from build123d import *

# Parameters (mm, degrees)
EXTRUDE_THIN1_DEPTH      = 3
EXTRUDE_THIN1_DEPTH_BACK = 3


with BuildPart() as part:
    # Sketch2 → Extrude-Thin1 (new, two sides)
    with BuildSketch(Plane.XY) as extrude_thin1_sk:
        with BuildLine():
            Line((-42.218873031, 27.812367004), (-33.426518735, 69.811728506))
            ThreePointArc((-33.426518735, 69.811728506), (7.206095545, 85.551006884), (5.054820151, 42.029676007))
            Line((5.054820151, 42.029676007), (-32.043042704, 20.465807333))
            ThreePointArc((-32.043042704, 20.465807333), (-39.516230782, 20.835209769), (-42.218873031, 27.812367004))
        make_face()
        with BuildLine():
            Line((-41.240090772, 27.60746388), (-32.447736476, 69.606825381))
            ThreePointArc((-32.447736476, 69.606825381), (6.620743822, 84.740227406), (4.552280795, 42.894230341))
            Line((4.552280795, 42.894230341), (-32.54558206, 21.330361667))
            ThreePointArc((-32.54558206, 21.330361667), (-38.93087906, 21.645989246), (-41.240090772, 27.60746388))
        make_face(mode=Mode.SUBTRACT)
    extrude(amount=EXTRUDE_THIN1_DEPTH)
    extrude(extrude_thin1_sk.sketch, amount=-EXTRUDE_THIN1_DEPTH_BACK)


solid = part.part
The model under review builds one solid part; all positions refer to its coordinate system, in mm. A direction names the side the tool comes from. Round coordinates to 2 decimals unless told otherwise and drop trailing zeros. Order: outer loops, then holes, each group sorted by start corner. A loop starts at its lowest first (then second) coordinate and runs counter-clockwise, first axis right, second up. Notation, with made-up numbers: (26.5, 76) -> (42.5, 76) arc R32 ccw to (42.5, 113) -> close; hole circle Ø10 at (54.5, -38). An arc over 180 degrees is marked (long way). Write item = value, one per line. Start each with the question number.
Item 1: Consider section A-A on y = 51. Write out the cut boundary in (x, z), plus the area to 3 significant figures.
Item 2: Mouldability with a two-part tool opening along Y and no side actions: class faces 3 (the face through (-13.23, 31.4, 0.04)), 4 (the face through (-1, 39, -3)), 5 (the face through (-13.74, 32.26, 0.04)) as released by +Y, released by -Y, zero draft, split by the parting line, or undercut.
Item 3: Consider section C-C on z = 1.85. Write out the cut boundary in (x, y).
Item 4: For line 1 along X through (y, z) = (76.5, -1.3); line 2 along Y through (x, z) = (-19, -2.35); line 3 along Y through (x, z) = (-8, -1.2), list the stretches that pass through material, from the lowest coordinate up.
Item 5: For faces 1 (the face through (-37.884, 48.518, 0.042)), 2 (the face through (-36.905, 48.313, 0.042)), list the 3-axis set-ups (+Z, -Z, +X, -X, +Y, -Y) from which the entire face can be reached by the end or side of a thin tool; tool diameter is ignored.
Item 6: Consider section B-B on x = -38. Write out the cut boundary in (y, z).
Item 7: Clearance check with a flat-ended pin moving along its axis: pin 1 Ø1 at (y, z) = (59.5, -2) entering from -X. State where the tip first meets the part, or that it passes through.
Conclusion:
q1.outline = (-37.36, -3) -> (-36.34, -3) -> (-36.34, 3) -> (-37.36, 3) -> close; (13.02, -3) -> (14.2, -3) -> (14.2, 3) -> (13.02, 3) -> close
q1.area = 13.2 mm2
q2.face_3 = released by -Y
q2.face_4 = zero draft
q2.face_5 = undercut
q3.outline = (-42.22, 27.81) arc R6.87 ccw to (-32.04, 20.47) -> (5.05, 42.03) arc R25.98 ccw (long way) to (-33.43, 69.81) -> close; hole (-41.24, 27.61) arc R5.87 ccw to (-32.55, 21.33) -> (4.55, 42.89) arc R24.98 ccw (long way) to (-32.45, 69.61) -> close
q4.line_1 = -31.03 to -29.9, 13.9 to 15.03
q4.line_2 = 28.05 to 29.2, 86.91 to 88.02
q4.line_3 = 34.44 to 35.6, 89.47 to 90.47
q5.face_1 = +Z, -Z, -X, +Y
q5.face_2 = +Z, -Z
q6.outline = (20.01, -3) -> (21.1, -3) -> (21.1, 3) -> (20.01, 3) -> close; (43.08, -3) -> (47.97, -3) -> (47.97, 3) -> (43.08, 3) -> close
q7.pin_1 = -35.69
